Can you work these out from the model? Positions are in its coordinate system, mm. A direction names the side the tool comes from. Give positions to 0.01 mm unless a question says otherwise; leave off trailing zeros. Order: outer loops, then holes, each group sorted by start corner. A loop starts at its lowest first (then second) coordinate and runs counter-clockwise, first axis right, second up. Notation, with made-up numbers: M 5.5,57.25 L 10.5,57.25 A21 cw 10.5,78.25 Z; hole C -22,63 d8. An arc over 180 degrees is marked long. Answer as a JSON object with one key per item and string values.
Autodesk Inventor part; units mm, degrees
ref_plane "YZ Plane" through (0, 0, 0) normal (1, 0, 0) x (0, 1, 0)
ref_plane "XZ Plane" through (0, 0, 0) normal (0, 1, 0) x (-1, 0, 0)
ref_plane "XY Plane" through (0, 0, 0) normal (0, 0, 1) x (1, 0, 0)
sketch "Sketch1" plane through (0, 0, 0) normal (0, 0, 1) x (1, 0, 0)
  line L0 (5.1012, -1.9833) -> (5.1012, -4.9833)
  line L1 (7.4512, -1.9833) -> (7.4512, 0.0167)
  line L2 (4.9512, 1.0167) -> (4.9512, -0.9833)
  line L3 (4.2012, 0.0167) -> (4.2012, -0.9833)
  line L4 (4.9512, 1.0167) -> (6.4512, 1.0167)
  line L5 (7.4512, -1.9833) -> (5.1012, -1.9833)
  line L6 (5.1012, -4.9833) -> (3.7012, -4.9833)
  line L7 (3.7012, -4.9833) -> (3.7012, 0.0167)
  line L8 (4.2012, -0.9833) -> (4.9512, -0.9833)
  line L9 (6.4512, 1.0167) -> (7.4512, 0.0167)
  line L10 (3.7012, 0.0167) -> (4.2012, 0.0167)
revolve "Revolution1" add sketch "Sketch1" angle 360 about axis through (3.7012, -4.9833, 0) along (0, 1, 0)
properties part number "MUSAB5" material "Bronze, Soft Tin"
1) I want a section at B-B on y = -3.55. Write out the boundary of the cut face in (x, z), and give its area (3 significant figures).
Results found:
{"outline": "C 3.7,0 d2.8", "area": "6.16 mm²"}
2) I'm going to push flat-ended pins straight in: pin 1 Ø1 at (x, y) = (2, 0) entering from -Z; pin 2 Ø0.5 at (x, z) = (3.5, 0) entering from +Y; pin 3 Ø1.5 at (y, z) = (-1, -1.5) entering from -X. Where does each tip first touch, or does it pass through?
Results found:
{"pin 1": "stops at z = -3.55", "pin 2": "stops at y = 0.02", "pin 3": "stops at x = 0.03"}
3) I need wall thicknesses on L1, parallel to X at y = -0.45, z = 0; L2, parallel to X at y = -2.6, z = 0; L3, parallel to Z at x = 3.75, y = -3.8. Which ranges of each line are inside material? Lowest first, please.
Results found:
{"L1": "x = -0.05 to 2.45, 3.2 to 4.2, 4.95 to 7.45", "L2": "x = 2.3 to 5.1", "L3": "z = -1.4 to 1.4"}
4) For faces 4 (the face through (5, 1.017, 1)), 5 (the face through (4.18, -0.49, 0.15)), which set-ups out of +Z, -Z, +X, -X, +Y, -Y let a thin tool reach every point of the face, with its end or its side?
Results found:
{"face 4": "+Z, -Z, +X, -X, +Y", "face 5": "+Y"}
5) Thinking about a two-plate mould opening in X: for faces 1 (the face through (4, 0.017, 0)), 2 (the face through (2.303, -3.504, 0.062)), 3 (the face through (4, -1.983, 2)), which applies, pulls with the +X half, pulls with the -X half, needs draft (parallel to the pull), parting line crosses it, or undercut?
Results found:
{"face 1": "undercut", "face 2": "parting line crosses it", "face 3": "needs draft"}
6) I want a section at A-A on z = 0. Write out the boundary of the cut face in (x, y).
Results found:
{"outline": "M -0.05,-1.98 L 2.3,-1.98 L 2.3,-4.98 L 5.1,-4.98 L 5.1,-1.98 L 7.45,-1.98 L 7.45,0.02 L 6.45,1.02 L 4.95,1.02 L 4.95,-0.98 L 4.2,-0.98 L 4.2,0.02 L 3.2,0.02 L 3.2,-0.98 L 2.45,-0.98 L 2.45,1.02 L 0.95,1.02 L -0.05,0.02 Z"}
